```python
from build123d import *

# Parameters (mm, degrees)
SKETCH1_R           = 9
SKETCH1_W           = 6
SKETCH1_H           = 6
SKETCH1_W_2         = 7.5
BOSS_EXTRUDE1_DEPTH = 6


with BuildPart() as part:
    # Sketch1 → Boss-Extrude1 (new body)
    with BuildSketch(Plane.XY):
        with BuildLine():
            ThreePointArc((20.5, 62.5), (13.075378798, 65.575378798), (10, 73))
            Line((10, 73), (-10, 73))
            Line((-10, 73), (-10, 83.5))
            Line((-10, 83.5), (-17.5, 83.5))
            Line((-17.5, 83.5), (-21, 83.5))
            Line((-21, 83.5), (-21, -83.5))
            Line((-21, -83.5), (-6, -83.5))
            Line((-6, -83.5), (0, -83.5))
            Line((0, -83.5), (6, -83.5))
            Line((6, -83.5), (21, -83.5))
            Line((21, -83.5), (21, 62.5))
            Line((21, 62.5), (20.5, 62.5))
        make_face()
        with Locations((0, -69.5)):
            Circle(SKETCH1_R, mode=Mode.SUBTRACT)
        with Locations((3, -86.5)):
            Rectangle(SKETCH1_W, SKETCH1_H)
        with Locations((-3, -86.5)):
            Rectangle(SKETCH1_W, SKETCH1_H)
        with Locations((-13.75, 86.5)):
            Rectangle(SKETCH1_W_2, SKETCH1_H)
    extrude(amount=-BOSS_EXTRUDE1_DEPTH)


solid = part.part
```
Could you check a few things on this model? Use its own coordinates, in mm. A direction names the side the tool comes from. Give positions to 0.01 mm unless a question says otherwise; leave off trailing zeros. Loops run counter-clockwise (first coordinate to the right, second up) from the corner with the lowest first, then second, coordinate; pieces in that order, holes last. Notation, with made-up numbers: (62.25, 53) - (71.25, 53) arc R10 cw to (71.25, 61) - close; hole circle Ø5 at (27, 57.25). An arc over 180 degrees is marked (long way). Use one line per item in the form item = value.
1. I want a section at B-B (z = -3.8). Please give me the cut outline in (x, y), and give its area (3 significant figures).
Response values:
outline = (-21, -83.5) - (-6, -83.5) - (-6, -89.5) - (6, -89.5) - (6, -83.5) - (21, -83.5) - (21, 62.5) - (20.5, 62.5) arc R10.5 cw to (10, 73) - (-10, 73) - (-10, 89.5) - (-17.5, 89.5) - (-17.5, 83.5) - (-21, 83.5) - close; hole circle Ø18 at (0, -69.5)
area = 6,460 mm²
2. I want a section at D-D (x = -13). Please give me the cut outline in (y, z).
Response values:
outline = (-83.5, -6) - (89.5, -6) - (89.5, 0) - (-83.5, 0) - close
3. I need wall thicknesses on probe 1 along Y at (x, z) = (0, -2.15); probe 2 along Y at (x, z) = (5, -2.1); probe 3 along Y at (x, z) = (-14, -3.7). Which ranges of each line are inside material? Lowest first, please.
Response values:
probe_1 = -89.5 to -78.5, -60.5 to 73
probe_2 = -89.5 to -76.98, -62.02 to 73
probe_3 = -83.5 to 89.5
4. I want a section at A-A (x = 0). Please give me the cut outline in (y, z), and give its area (3 significant figures).
Response values:
outline = (-89.5, -6) - (-78.5, -6) - (-78.5, 0) - (-89.5, 0) - close; (-60.5, -6) - (73, -6) - (73, 0) - (-60.5, 0) - close
area = 867 mm²
5. I want a section at C-C (y = -69.5). Please give me the cut outline in (x, z), and give its area (3 significant figures).
Response values:
outline = (-21, -6) - (-9, -6) - (-9, 0) - (-21, 0) - close; (9, -6) - (21, -6) - (21, 0) - (9, 0) - close
area = 144 mm²
6. Thinking about a two-plate mould opening in Y: for faces 1 (the face through (-10, 81, -3)), 2 (the face through (-19, 83.5, -3)), 3 (the face through (-1.951, -78.286, -2.958)), which applies, released by +Y, released by -Y, zero draft, split by the parting line, or undercut?
Response values:
face_1 = zero draft
face_2 = released by +Y
face_3 = undercut
7. On a 3-axis mill with a long thin cutter (end or side, diameter ignored), from which of +Z, -Z, +X, -X, +Y, -Y can I reach the whole of each face in a straight line? I mean faces 4 (the face through (13, -83.5, -3)), 5 (the face through (0, 73, -3)), 6 (the face through (-14, -83.5, -3)), 7 (the face through (-17.5, 86, -3)). Say none if no direction works.
Response values:
face_4 = +Z, -Z, +X, -Y
face_5 = +Z, -Z, +X, +Y
face_6 = +Z, -Z, -X, -Y
face_7 = +Z, -Z, -X, +Y
8. I'm going to push flat-ended pins straight in: pin 1 Ø2 at (x, z) = (14, -4) entering from +Y; pin 2 Ø1.8 at (y, z) = (-85.5, -3) entering from +X; pin 3 Ø1.8 at (x, z) = (-19.5, -3.5) entering from +Y. Where does each tip first touch, or does it pass through?
Response values:
pin_1 = 65.65
pin_2 = 6
pin_3 = 83.5
